Here's how the part is built. I have some questions about the finished solid (model axes, mm). A direction names the side the tool comes from. Coordinates: 2 decimals unless noted, no trailing zeros. Write each loop counter-clockwise with the first axis right and the second up, starting at its lowest first coordinate (ties: lowest second). Pieces come first, ordered by that corner, then holes. Notation, with made-up numbers: (32, 54) -> (82, 54) arc R23 ccw to (82, 91) -> close; hole circle Ø8 at (2, 5.5). An arc over 180 degrees is marked (long way). Put each result on its own line as item: value. Start each with the question number.
Item 1: For pin 1 (1 mm diameter, centred on y = -3.5, z = 7, fed in from +X); pin 2 (1.9 mm diameter, centred on x = -0.5, y = -0.5, fed in from +Z); pin 3 (1 mm diameter, centred on y = 12, z = 8.5, fed in from +X), each with a flat end and sliding along its axis, tell me the tip position at first contact or that it passes through.
Item 2: I want a section at A-A, the plane x = 0. List the corners of the cut face in (y, z) for me.
Item 3: I want a section at C-C, the plane z = 21. List the corners of the cut face in (x, y) for me.
Item 4: I want a section at D-D, the plane x = -13.5. List the corners of the cut face in (y, z) for me, then the cut area to 3 significant figures.
Item 5: If we mould it in two halves opening along Y, with no side actions, what happens to faces 3 (the face through (2, -4, 10)), 4 (the face through (-2, -19, 40)), 5 (the face through (-4.97, -22.38, 19.72))? For each: released by +Y, released by -Y, zero draft, split by the parting line, or undercut.
Item 6: On a 3-axis mill with a long thin cutter (end or side, diameter ignored), from which of +Z, -Z, +X, -X, +Y, -Y can I reach the whole of each face in a straight line? I mean faces 1 (the face through (-1.183, -5.327, 8.986)), 2 (the face through (0, 0, 0)). Say none if no direction works.
Item 7: I need wall thicknesses on line 1 (Y direction, x = 0, z = 26); line 2 (Z direction, x = 2.5, y = 13); line 3 (X direction, y = -3.5, z = 12). Which ranges of each line are inside material? Lowest first, please. Write a range as [from, to].
from build123d import *

# Parameters (mm, degrees)
SKETCH_R     = 22.925405
PAD_DEPTH    = 40
SKETCH001_R  = 18.304244
POCKET_DEPTH = 32
SKETCH002_R  = 5.45658
PAD001_DEPTH = 2
SKETCH003_R  = 4.228884
PAD002_DEPTH = 20
FILLET_R     = 1


with BuildPart() as part:
    # Sketch → Pad (new body)
    with BuildSketch(Plane.XY):
        Circle(SKETCH_R)
    extrude(amount=PAD_DEPTH)

    # Sketch001 (on Face3 of Pad) → Pocket (cut)
    with BuildSketch(Plane.XY.offset(40)):
        Circle(SKETCH001_R)
    extrude(amount=-POCKET_DEPTH, mode=Mode.SUBTRACT)

    # Sketch002 (on Face5 of Pocket) → Pad001 (join)
    with BuildSketch(Plane.XY.offset(8)):
        Circle(SKETCH002_R)
    extrude(amount=PAD001_DEPTH)

    # Sketch003 (on Face7 of Pad001) → Pad002 (join)
    with BuildSketch(Plane.XY.offset(10)):
        Circle(SKETCH003_R)
    extrude(amount=PAD002_DEPTH)

    # Fillet
    fillet_edges = [part.edges().sort_by_distance(p)[0] for p in [
        (-4.228884, 0, 30),
    ]]
    fillet(fillet_edges, radius=FILLET_R)


solid = part.part
Calculated:
1. pin 1: stops at x = 22.73
1. pin 2: stops at z = 30
1. pin 3: stops at x = 19.83
2. outline: (-22.93, 0) -> (22.93, 0) -> (22.93, 40) -> (18.3, 40) -> (18.3, 8) -> (5.46, 8) -> (5.46, 10) -> (4.23, 10) -> (4.23, 29) arc R1 ccw to (3.23, 30) -> (-3.23, 30) arc R1 ccw to (-4.23, 29) -> (-4.23, 10) -> (-5.46, 10) -> (-5.46, 8) -> (-18.3, 8) -> (-18.3, 40) -> (-22.93, 40) -> close
3. outline: circle Ø45.85 at (0, 0); circle Ø8.46 at (0, 0); hole circle Ø36.61 at (0, 0)
4. outline: (-18.53, 0) -> (18.53, 0) -> (18.53, 40) -> (12.36, 40) -> (12.36, 8) -> (-12.36, 8) -> (-12.36, 40) -> (-18.53, 40) -> close
4. area: 691 mm2
5. face 3: undercut
5. face 4: zero draft
5. face 5: split by the parting line
6. face 1: +Z
6. face 2: -Z, +X, -X, +Y, -Y
7. line 1: y = [-22.93, -18.3], [-4.23, 4.23], [18.3, 22.93]
7. line 2: z = [0, 8]
7. line 3: x = [-22.66, -17.97], [-2.37, 2.37], [17.97, 22.66]
